Solid Edge part; units mm, degrees
sketch "Sketch1" plane through (0, 0, 0) normal (0, 0, 1) x (1, 0, 0)
  line L0 (6.0091, 30.5) -> (6.0091, 21.1635)
  line L1 (22.0001, 0) -> (22.0001, -21.9937)
  line L2 (-0.5256, -21.9937) -> (22.0001, -21.9937)
  line L3 (-0.5256, -21.9937) -> (-21.9999, -21.9937)
  line L4 (-21.9999, 0) -> (-21.9999, -21.9937)
  arc A0 (-21.9999, 0) -> (-4.9909, 21.4264) centre (0.0001, 0) cw
  line L5 (-4.9909, 30.5) -> (-4.9909, 21.4264)
  line L6 (0.0091, 30.5) -> (-4.9909, 30.5)
  line L7 (0.0091, 20.5) -> (0.0091, 30.5)
  line L8 (1.0091, 20.5) -> (1.0091, 20.4752)
  line L9 (1.0091, 20.5) -> (1.0091, 30.5)
  line L10 (1.0091, 30.5) -> (6.0091, 30.5)
  arc A1 (6.0091, 21.1635) -> (22.0001, 0) centre (0.0001, 0) cw
  arc A2 (1.0091, 20.4752) -> (0.0091, 20.5) centre (0.0001, 0) cw
extrude "Protrusion1" add sketch "Sketch1" along normal blind 30
hole "Hole_1" at (-4.9909, 25.9632, 7.4167) direction (1, 0, 0) diameter 6.35 end up to next
hole "Hole1" at (-4.9909, 25.9359, 21.8715) direction (1, 0, 0) diameter 6.35 end up to next
hole "Hole_3" at (1.0091, 25.9256, 7.4167) direction (1, 0, 0) diameter 6.35 end up to next
hole "Hole2" at (1.0091, 25.9256, 21.8167) direction (1, 0, 0) diameter 6.35 end up to next
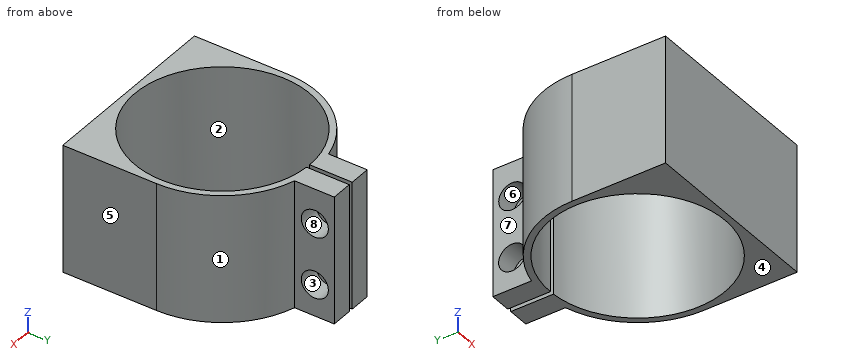
For this review, take the finished solid that the model builds, in its own axes (mm). Face numbers are marked on the shaded views. A direction names the side the tool comes from. Give positions to 0.01 mm unless a question says otherwise; leave off trailing zeros. Write each loop counter-clockwise with the first axis right and the second up, starting at its lowest first coordinate (ties: lowest second). Pieces come first, ordered by that corner, then holes. Notation, with made-up numbers: M -16,63.5 L 2,63.5 A7 ccw 2,68.5 Z; hole C -13,89.25 d1. An arc over 180 degrees is marked long. Answer as a JSON object with one key per item and string values. Group by question number.
Item 1: For probe 1 along X at (y, z) = (25, 2); probe 2 along X at (y, z) = (10, 16); probe 3 along Y at (x, z) = (-4.5, 28), list the stretches that pass through material, from the lowest coordinate up. Write a range as [from, to].
Item 2: For pin 1 Ø1 at (x, y) = (16.5, 8.5) entering from -Z; pin 2 Ø3 at (y, z) = (24, 10) entering from +X; pin 3 Ø10.5 at (y, z) = (25, 16) entering from +X; pin 4 Ø8 at (y, z) = (24, 20.5) entering from -X, all flat-tipped, find the tip position at first contact; note any pin that passes through.
Item 3: Consider section B-B on x = -2. Count the separate pieces of the cut face and the enclosed holes in it, plus the area to 3 significant figures.
Item 4: Consider section D-D on x = -11.5. Write out the cut boundary in (y, z).
Item 5: Consider section A-A on y = 2. Write out the cut boundary in (x, z).
Item 6: Draft analysis for pull direction Y (two halves, no side actions). For the marked faces 1, 2, 3 and 4, state which applies: +Y half, -Y half, draft (parallel to the pull), parting line (faces both ways), or undercut.
Item 7: Tool access review of the marked faces 5, 6, 7 and 8: name each direction out of +Z, -Z, +X, -X, +Y, -Y from which nothing blocks a thin tool from reaching the whole face with its end or side.
Check result:
{
 "1": {"probe 1": "x = [-4.99, 0.01], [1.01, 6.01]", "probe 2": "x = [-19.6, -17.9], [17.9, 19.6]", "probe 3": "y = [-21.99, -20], [20, 30.5]"},
 "2": {"pin 1": "passes through", "pin 2": "stops at x = 6.01", "pin 3": "stops at x = 9.69", "pin 4": "stops at x = -9.17"},
 "3": {"separate pieces": "2", "enclosed holes": "2", "area": "287 mm^2"},
 "4": {"outline": "M -21.99,0 L -16.97,0 L -16.97,30 L -21.99,30 Z; M 16.97,0 L 18.75,0 L 18.75,30 L 16.97,30 Z"},
 "5": {"outline": "M -21.91,0 L -20.4,0 L -20.4,30 L -21.91,30 Z; M 20.4,0 L 21.91,0 L 21.91,30 L 20.4,30 Z"},
 "6": {"face 1": "+Y half", "face 2": "undercut", "face 3": "undercut", "face 4": "draft"},
 "7": {"face 5": "+Z, -Z, +X, +Y, -Y", "face 6": "-X", "face 7": "+Z, -Z, -X, +Y", "face 8": "+X"}
}
